from build123d import *

# Parameters (mm, degrees)
F1_DEPTH = 25


with BuildPart() as f1:
    # F0 (on Top) → F1 (new body)
    with BuildSketch(Plane.XY):
        with BuildLine():
            ThreePointArc((29.813631, -39.158033), (35, -39.5), (40.186369, -39.158033))
            Line((40.186369, -39.158033), (41.516062, -29.2838))
            ThreePointArc((41.516062, -29.2838), (46.480503, -27.716386), (51.099222, -25.314325))
            Line((51.099222, -25.314325), (59.021594, -31.356228))
            ThreePointArc((59.021594, -31.356228), (62.930718, -27.930718), (66.356228, -24.021594))
            Line((66.356228, -24.021594), (60.314325, -16.099222))
            ThreePointArc((60.314325, -16.099222), (62.716386, -11.480503), (64.2838, -6.516062))
            Line((64.2838, -6.516062), (74.158033, -5.186369))
            ThreePointArc((74.158033, -5.186369), (74.5, 0), (74.158033, 5.186369))
            Line((74.158033, 5.186369), (64.2838, 6.516062))
            ThreePointArc((64.2838, 6.516062), (62.716386, 11.480503), (60.314325, 16.099222))
            Line((60.314325, 16.099222), (66.356228, 24.021594))
            ThreePointArc((66.356228, 24.021594), (62.930718, 27.930718), (59.021594, 31.356228))
            Line((59.021594, 31.356228), (51.099222, 25.314325))
            ThreePointArc((51.099222, 25.314325), (46.480503, 27.716386), (41.516062, 29.2838))
            Line((41.516062, 29.2838), (40.186369, 39.158033))
            ThreePointArc((40.186369, 39.158033), (35, 39.5), (29.813631, 39.158033))
            Line((29.813631, 39.158033), (28.483938, 29.2838))
            ThreePointArc((28.483938, 29.2838), (23.519497, 27.716386), (18.900778, 25.314325))
            Line((18.900778, 25.314325), (10.978406, 31.356228))
            ThreePointArc((10.978406, 31.356228), (7.069282, 27.930718), (3.643772, 24.021594))
            Line((3.643772, 24.021594), (9.685675, 16.099222))
            ThreePointArc((9.685675, 16.099222), (7.283614, 11.480503), (5.7162, 6.516062))
            Line((5.7162, 6.516062), (-4.158033, 5.186369))
            ThreePointArc((-4.158033, 5.186369), (-4.5, 0), (-4.158033, -5.186369))
            Line((-4.158033, -5.186369), (5.7162, -6.516062))
            ThreePointArc((5.7162, -6.516062), (7.283614, -11.480503), (9.685675, -16.099222))
            Line((9.685675, -16.099222), (3.643772, -24.021594))
            ThreePointArc((3.643772, -24.021594), (7.069282, -27.930718), (10.978406, -31.356228))
            Line((10.978406, -31.356228), (18.900778, -25.314325))
            ThreePointArc((18.900778, -25.314325), (23.519497, -27.716386), (28.483938, -29.2838))
            Line((28.483938, -29.2838), (29.813631, -39.158033))
        make_face()
    extrude(amount=F1_DEPTH)


solid = f1.part
Could you check a few things on this model? Use its own coordinates, in mm. A direction names the side the tool comes from. Coordinates: 2 decimals unless noted, no trailing zeros. Loops run counter-clockwise (first coordinate to the right, second up) from the corner with the lowest first, then second, coordinate; pieces in that order, holes last.
1. Imagine slicing it at B-B (y = 26.5). Please give me the cut outline in (x, z), and give its area (4 significant figures).
2. For P1, Ø8, axis at x = 26.5, z = 11, coming from the -Y side; P2, Ø1, axis at x = 7.5, z = 17.5, coming from the +Y side, each with a flat end and sliding along its axis, tell me the tip position at first contact or that it passes through.
3. I need wall thicknesses on L1, parallel to X at y = -26, z = 9; L2, parallel to X at y = -25.5, z = 7; L3, parallel to Y at x = 61, z = 2.25. Which ranges of each line are inside material? Lowest first, please.
4. For faces 1 (the face through (0.71, -5.84, 12.32)), 2 (the face through (69.29, 5.84, 12.32)), 3 (the face through (23.587, 27.744, 12.325)), which set-ups out of +Z, -Z, +X, -X, +Y, -Y let a thin tool reach every point of the face, with its end or its side?
5. We'd pull the mould along Y, two halves only. Please class faces 4 (the face through (6.71, -20, 12.32)), 5 (the face through (34, 1, 25)), 6 (the face through (55, -28.29, 12.32)): released by +Y, released by -Y, zero draft, split by the parting line, or undercut.
6. Imagine slicing it at D-D (y = -11). Please give me the cut outline in (x, z).
7. Imagine slicing it at C-C (x = 53.5). Please give me the cut outline in (y, z), and give its area (3 significant figures).
Computed values:
1. outline: (5.71, 0) - (17.35, 0) - (17.35, 25) - (5.71, 25) - close; (20.94, 0) - (49.06, 0) - (49.06, 25) - (20.94, 25) - close; (52.65, 0) - (64.29, 0) - (64.29, 25) - (52.65, 25) - close
1. area: 1,285 mm2
2. P1: stops at y = -39.24
2. P2: stops at y = 28.83
3. L1: x = 5.26 to 18, 20.03 to 49.97, 52 to 64.74
3. L2: x = 4.83 to 18.66, 19.2 to 50.8, 51.34 to 65.17
3. L3: y = -29.74 to -17, -14.97 to 14.97, 17 to 29.74
4. face 1: +Z, -Z, -X
4. face 2: +Z, -Z, +X
4. face 3: +Z, -Z, +Y
5. face 4: undercut
5. face 5: zero draft
5. face 6: released by -Y
6. outline: (7.09, 0) - (62.91, 0) - (62.91, 25) - (7.09, 25) - close
7. outline: (-27.15, 0) - (27.15, 0) - (27.15, 25) - (-27.15, 25) - close
7. area: 1,360 mm2
